Design review of the part built by this model. Coordinates are the model's own, in mm. Give positions to 0.01 mm unless a question says otherwise; leave off trailing zeros. Loops run counter-clockwise (first coordinate to the right, second up) from the corner with the lowest first, then second, coordinate; pieces in that order, holes last. Notation, with made-up numbers: (58, 74) -> (89, 74) arc R12 ccw to (89, 84) -> close; hole circle Ø5 at (11.25, -19). An arc over 180 degrees is marked (long way). Use a Markdown table: item, result. Add a question column.
1. For pin 1 Ø4 at (x, z) = (-0.5, 168.5) entering from +Y; pin 2 Ø5 at (x, z) = (-1, 126.5) entering from +Y, all flat-tipped, find the tip position at first contact; note any pin that passes through.
2. Add section B-B (z = 93). State the section outline as (x, y) points.
3. Add section A-A (y = 2.25). Count the separate pieces of the cut face and the enclosed holes in it, and give its area (3 significant figures).
4. To check wall thickness, follow line 1 (X direction, y = -2.05, z = 187.5); line 2 (Y direction, x = 3, z = 27.5); line 3 (X direction, y = 1.25, z = 27.5). State the ranges of each line that lie inside material, in increasing order.
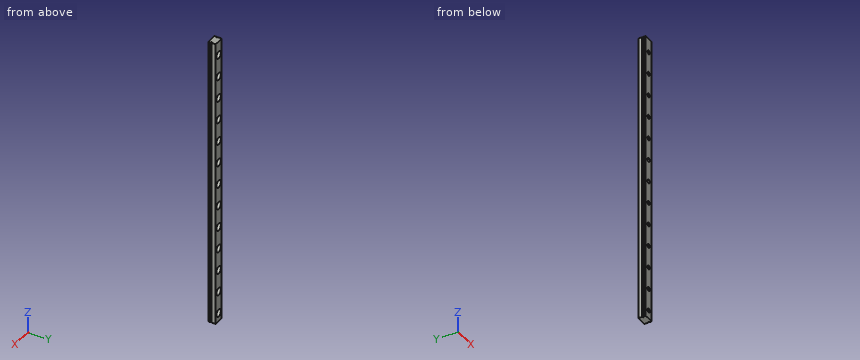
```python
from build123d import *

# Parameters (mm, degrees)
SKETCH_1_W          = 9
SKETCH_1_H          = 6.5
EXTRUDE_1_DEPTH     = 260
SKETCH_2_R          = 1.75
CUT_EXTRUDE_1_DEPTH = 7.5
SKETCH_3_R          = 3.25
CUT_EXTRUDE_2_DEPTH = 3.5
CUT_EXTRUDE_3_DEPTH = 261


with BuildPart() as part:
    # 草图1 → 凸台-拉伸1 (new body)
    with BuildSketch(Plane.XY):
        Rectangle(SKETCH_1_W, SKETCH_1_H)
    extrude(amount=EXTRUDE_1_DEPTH)

    # 草图2 → 切除-拉伸1 (cut, through all)
    with BuildSketch(Plane(origin=(0, 3.25, 0), x_dir=(1, 0, 0), z_dir=(0, 1, 0))):
        with Locations((0, -7.5)):
            Circle(SKETCH_2_R)
        with Locations((0, -27.5)):
            Circle(SKETCH_2_R)
        with Locations((0, -47.5)):
            Circle(SKETCH_2_R)
        with Locations((0, -67.5)):
            Circle(SKETCH_2_R)
        with Locations((0, -87.5)):
            Circle(SKETCH_2_R)
        with Locations((0, -107.5)):
            Circle(SKETCH_2_R)
        with Locations((0, -127.5)):
            Circle(SKETCH_2_R)
        with Locations((0, -147.5)):
            Circle(SKETCH_2_R)
        with Locations((0, -167.5)):
            Circle(SKETCH_2_R)
        with Locations((0, -187.5)):
            Circle(SKETCH_2_R)
        with Locations((0, -207.5)):
            Circle(SKETCH_2_R)
        with Locations((0, -227.5)):
            Circle(SKETCH_2_R)
        with Locations((0, -247.5)):
            Circle(SKETCH_2_R)
        with Locations((0, -267.5)):
            Circle(SKETCH_2_R)
        with Locations((0, -287.5)):
            Circle(SKETCH_2_R)
        with Locations((0, -307.5)):
            Circle(SKETCH_2_R)
        with Locations((0, -327.5)):
            Circle(SKETCH_2_R)
        with Locations((0, -347.5)):
            Circle(SKETCH_2_R)
        with Locations((0, -367.5)):
            Circle(SKETCH_2_R)
        with Locations((0, -387.5)):
            Circle(SKETCH_2_R)
    extrude(amount=-CUT_EXTRUDE_1_DEPTH, mode=Mode.SUBTRACT)

    # 草图3 → 切除-拉伸2 (cut)
    with BuildSketch(Plane(origin=(0, 3.25, 0), x_dir=(1, 0, 0), z_dir=(0, 1, 0))):
        with Locations((0, -7.5)):
            Circle(SKETCH_3_R)
        with Locations((0, -27.5)):
            Circle(SKETCH_3_R)
        with Locations((0, -47.5)):
            Circle(SKETCH_3_R)
        with Locations((0, -67.5)):
            Circle(SKETCH_3_R)
        with Locations((0, -87.5)):
            Circle(SKETCH_3_R)
        with Locations((0, -107.5)):
            Circle(SKETCH_3_R)
        with Locations((0, -127.5)):
            Circle(SKETCH_3_R)
        with Locations((0, -147.5)):
            Circle(SKETCH_3_R)
        with Locations((0, -167.5)):
            Circle(SKETCH_3_R)
        with Locations((0, -187.5)):
            Circle(SKETCH_3_R)
        with Locations((0, -207.5)):
            Circle(SKETCH_3_R)
        with Locations((0, -227.5)):
            Circle(SKETCH_3_R)
        with Locations((0, -247.5)):
            Circle(SKETCH_3_R)
        with Locations((0, -267.5)):
            Circle(SKETCH_3_R)
        with Locations((0, -287.5)):
            Circle(SKETCH_3_R)
        with Locations((0, -307.5)):
            Circle(SKETCH_3_R)
        with Locations((0, -327.5)):
            Circle(SKETCH_3_R)
        with Locations((0, -347.5)):
            Circle(SKETCH_3_R)
        with Locations((0, -367.5)):
            Circle(SKETCH_3_R)
        with Locations((0, -387.5)):
            Circle(SKETCH_3_R)
    extrude(amount=-CUT_EXTRUDE_2_DEPTH, mode=Mode.SUBTRACT)

    # 草图4 → 切除-拉伸3 (cut, through all)
    with BuildSketch(Plane(origin=(0, 0, 0), x_dir=(-1, 0, 0), z_dir=(0, 0, -1))):
        Polygon((4.5, -0.25), (3.5, -0.45), (3.5, -1.05), (4.5, -1.25), align=None)
        Polygon((-4.5, -0.25), (-3.5, -0.45), (-3.5, -1.05), (-4.5, -1.25), align=None)
    extrude(amount=-CUT_EXTRUDE_3_DEPTH, mode=Mode.SUBTRACT)


solid = part.part
```
Taken from the geometry:
| question | item | result |
|---|---|---|
| 1 | pin 1 | stops at y = -0.25 |
| 1 | pin 2 | stops at y = 3.25 |
| 2 | outline | (-4.5, -3.25) -> (4.5, -3.25) -> (4.5, -1.25) -> (3.5, -1.05) -> (3.5, -0.45) -> (4.5, -0.25) -> (4.5, 3.25) -> (-4.5, 3.25) -> (-4.5, -0.25) -> (-3.5, -0.45) -> (-3.5, -1.05) -> (-4.5, -1.25) -> close |
| 3 | separate pieces | 1 |
| 3 | enclosed holes | 13 |
| 3 | area | 1,910 mm^2 |
| 4 | line 1 | x = -4.5 to -1.75, 1.75 to 4.5 |
| 4 | line 2 | y = -3.25 to -0.25 |
| 4 | line 3 | x = -4.5 to -3.25, 3.25 to 4.5 |
